For this review, take the finished solid that the model builds, in its own axes (mm). A direction names the side the tool comes from. Coordinates: 2 decimals unless noted, no trailing zeros. Order: outer loops, then holes, each group sorted by start corner. A loop starts at its lowest first (then second) coordinate and runs counter-clockwise, first axis right, second up.
from build123d import *

# Parameters (mm, degrees)
CROQUIS1_W                                  = 100
CROQUIS1_H                                  = 50
SALIENTE_EXTRUIR1_DEPTH                     = 5
SALIENTE_EXTRUIR2_DEPTH                     = 40
CROQUIS3_W                                  = 95
CROQUIS3_H                                  = 2
CORTAR_EXTRUIR1_DEPTH                       = 2
CROQUIS4_W                                  = 95
CROQUIS4_H                                  = 2
CORTAR_EXTRUIR2_DEPTH                       = 2
DI_METRO_DE_TALADRO_2_0_2_1_D               = 2
DI_METRO_DE_TALADRO_2_0_2_2_D               = 2
DI_METRO_DE_TALADRO_2_0_2_2_DEPTH           = 10
DI_METRO_DE_TALADRO_2_0_2_2_TIP             = 0.600860619
DI_METRO_DE_TALADRO_2_0_2_2_ON_FACE_2_D     = 2
DI_METRO_DE_TALADRO_2_0_2_2_ON_FACE_2_DEPTH = 10
DI_METRO_DE_TALADRO_2_0_2_2_ON_FACE_2_TIP   = 0.600860619


with BuildPart() as part:
    # Croquis1 → Saliente-Extruir1 (new body)
    with BuildSketch(Plane(origin=(0, 0, 0), x_dir=(1, 0, 0), z_dir=(0, 1, 0))):
        with Locations((50, 25)):
            Rectangle(CROQUIS1_W, CROQUIS1_H)
    extrude(amount=SALIENTE_EXTRUIR1_DEPTH)

    # Croquis2 → Saliente-Extruir2 (add)
    with BuildSketch(Plane(origin=(0, 5, 0), x_dir=(1, 0, 0), z_dir=(0, 1, 0))):
        Polygon((0, 45), (95, 45), (95, 0), (100, 0), (100, 50), (0, 50), align=None)
    extrude(amount=SALIENTE_EXTRUIR2_DEPTH)

    # Croquis3 → Cortar-Extruir1 (cut)
    with BuildSketch(Plane.XY.offset(-45)):
        with Locations((47.5, 42.5)):
            Rectangle(CROQUIS3_W, CROQUIS3_H)
    extrude(amount=-CORTAR_EXTRUIR1_DEPTH, mode=Mode.SUBTRACT)

    # Croquis4 → Cortar-Extruir2 (cut)
    with BuildSketch(Plane(origin=(0, 5, 0), x_dir=(1, 0, 0), z_dir=(0, 1, 0))):
        with Locations((47.5, 2.5)):
            Rectangle(CROQUIS4_W, CROQUIS4_H)
    extrude(amount=-CORTAR_EXTRUIR2_DEPTH, mode=Mode.SUBTRACT)

    # Diámetro de taladro Ø2.0 (2)1 (through all)
    with Locations(Plane(origin=(95, 42.5, -42.5), x_dir=(0, 0, -1), z_dir=(-1, 0, 0))):
        with Locations((0, 0), (-40, 35)):
            Hole(DI_METRO_DE_TALADRO_2_0_2_1_D / 2)

    # Diámetro de taladro Ø2.0 (2)2
    with Locations(Plane(origin=(2.5, 37.5, -50), x_dir=(-1, 0, 0), z_dir=(0, 0, -1))):
        with Locations((0, 0)):
            Hole(DI_METRO_DE_TALADRO_2_0_2_2_D / 2, depth=DI_METRO_DE_TALADRO_2_0_2_2_DEPTH)
            with Locations((0, 0, -(DI_METRO_DE_TALADRO_2_0_2_2_DEPTH + DI_METRO_DE_TALADRO_2_0_2_2_TIP / 2))):  # 118° drill point
                Cone(0, DI_METRO_DE_TALADRO_2_0_2_2_D / 2, DI_METRO_DE_TALADRO_2_0_2_2_TIP, mode=Mode.SUBTRACT)

    # Diámetro de taladro Ø2.0 (2)2 on face 2
    with Locations(Plane(origin=(2.5, 0, -7.5), x_dir=(0, 0, -1), z_dir=(0, -1, 0))):
        with Locations((0, 0)):
            Hole(DI_METRO_DE_TALADRO_2_0_2_2_ON_FACE_2_D / 2, depth=DI_METRO_DE_TALADRO_2_0_2_2_ON_FACE_2_DEPTH)
            with Locations((0, 0, -(DI_METRO_DE_TALADRO_2_0_2_2_ON_FACE_2_DEPTH + DI_METRO_DE_TALADRO_2_0_2_2_ON_FACE_2_TIP / 2))):  # 118° drill point
                Cone(0, DI_METRO_DE_TALADRO_2_0_2_2_ON_FACE_2_D / 2, DI_METRO_DE_TALADRO_2_0_2_2_ON_FACE_2_TIP, mode=Mode.SUBTRACT)


solid = part.part
1. To check wall thickness, follow L1, parallel to Z at x = 96.9, y = 7.5; L2, parallel to Y at x = 79, z = -23; L3, parallel to X at y = 32, z = -37.5. State the ranges of each line that lie inside material, in increasing order.
Answer below:
L1: z = -50 to -3.5, -1.5 to 0
L2: y = 0 to 5
L3: x = 95 to 100
2. The part is to be moulded in two halves that separate along Y. For faces 6 (the face through (47, 23, -45)), 7 (the face through (47, 41.5, -46)), 8 (the face through (47, 3, -3)), say which applies: +Y half, -Y half, draft (parallel to the pull), parting line (faces both ways), or undercut.
Answer below:
face 6: draft
face 7: undercut
face 8: +Y half
3. Take a section at D-D, the plane x = 35. Give the boundary of the cut face in (y, z), plus the area to 3 significant figures.
Answer below:
outline: (0, -50) - (45, -50) - (45, -45) - (43.5, -45) - (43.5, -47) - (41.5, -47) - (41.5, -45) - (5, -45) - (5, -3.5) - (3, -3.5) - (3, -1.5) - (5, -1.5) - (5, 0) - (0, 0) - close
area: 442 mm2
4. Take a section at C-C, the plane x = 2.5. Give the boundary of the cut face in (y, z).
Answer below:
outline: (0, -50) - (36.5, -50) - (36.5, -45) - (5, -45) - (5, -8.5) - (0, -8.5) - close; (0, -6.5) - (5, -6.5) - (5, -3.5) - (3, -3.5) - (3, -1.5) - (5, -1.5) - (5, 0) - (0, 0) - close; (38.5, -50) - (45, -50) - (45, -45) - (43.5, -45) - (43.5, -47) - (41.5, -47) - (41.5, -45) - (38.5, -45) - close
5. Take a section at B-B, the plane y = 37.5. Give the boundary of the cut face in (x, z), plus the area to 3 significant figures.
Answer below:
outline: (0, -50) - (1.5, -50) - (1.5, -45) - (0, -45) - close; (3.5, -50) - (100, -50) - (100, 0) - (95, 0) - (95, -45) - (3.5, -45) - close
area: 715 mm2
6. Clearance check with flat-ended pins moving along their axes: pin 1 Ø10 at (x, z) = (70, -28.5) entering from -Y; pin 2 Ø1.5 at (x, z) = (36, -27) entering from +Y; pin 3 Ø1.2 at (y, z) = (7.5, -2.5) entering from -X; pin 4 Ø3 at (x, y) = (73, 40) entering from +Z. State where each tip first meets the part, or that it passes through.
Answer below:
pin 1: stops at y = 0
pin 2: stops at y = 5
pin 3: passes through
pin 4: stops at z = -45
7. Take a section at A-A, the plane z = -2.5. Give the boundary of the cut face in (x, y).
Answer below:
outline: (0, 0) - (100, 0) - (100, 6.5) - (95, 6.5) - (95, 3) - (0, 3) - close; (95, 8.5) - (100, 8.5) - (100, 45) - (95, 45) - close
8. Machinability: for faces 1 (the face through (47, 43.5, -46)), 2 (the face through (47, 4, -1.5)), 3 (the face through (47, 5, -25)), 4 (the face through (49, 0, -25)), 5 (the face through (57, 4, 0)), which of the approach directions +Z, -Z, +X, -X, +Y, -Y give a long, thin tool a straight path to every point of the face, cutting with its end or side? Answer none if there is none.
Answer below:
face 1: +Z, -X
face 2: -X, +Y
face 3: +Z, -X, +Y
face 4: +Z, -Z, +X, -X, -Y
face 5: +Z, +X, -X, +Y, -Y
